Geometry: final body of the model. Coordinates: model frame, mm. A direction names the side the tool comes from. Coordinates: 2 decimals unless noted, no trailing zeros. Order: outer loops, then holes, each group sorted by start corner. A loop starts at its lowest first (then second) coordinate and runs counter-clockwise, first axis right, second up. Notation, with made-up numbers: (63.25, 54) - (86.25, 54) arc R13 ccw to (86.25, 73) - close; hole circle Ø11 at (45, 75.25). An arc over 180 degrees is marked (long way). Use a Markdown table: item, result. Add a question column.
```python
from build123d import *

# Parameters (mm, degrees)
SKETCH1_W                      = 174
SKETCH1_H                      = 50
BOSS_EXTRUDE1_DEPTH            = 13
M6_CLEARANCE_HOLE1_D           = 6.6
M6_CLEARANCE_HOLE1_CSINK_D     = 6.65
M6_CLEARANCE_HOLE1_CSINK_ANGLE = 100
SKETCH6_W                      = 80
SKETCH6_H                      = 13
BOSS_EXTRUDE2_DEPTH            = 40
SKETCH7_W                      = 80
SKETCH7_H                      = 40
BOSS_EXTRUDE3_DEPTH            = 50
CUT_EXTRUDE2_DEPTH             = 120.557517539
CUT_EXTRUDE2_DEPTH_BACK        = 120.557517539
SKETCH9_R                      = 14.29
M6_CLEARANCE_HOLE2_AT_2_COUNT  = 2
M6_CLEARANCE_HOLE2_AT_2_PITCH  = 37.540299013
M6_CLEARANCE_HOLE2_AT_3_COUNT  = 2
M6_CLEARANCE_HOLE2_AT_3_PITCH  = 37.540299013
M6_CLEARANCE_HOLE2_AT_4_COUNT  = 2
M6_CLEARANCE_HOLE2_AT_4_PITCH  = 53.09
CUT_EXTRUDE3_DEPTH             = 6.93
CUT_EXTRUDE3_DEPTH_BACK        = 6.93
SKETCH17_W                     = 28.58
SKETCH17_H                     = 29
CUT_EXTRUDE4_DEPTH             = 135.792433022
CUT_EXTRUDE5_DEPTH             = 50


with BuildPart() as part:
    # Sketch1 → Boss-Extrude1 (new body)
    with BuildSketch(Plane(origin=(0, 0, 0), x_dir=(1, 0, 0), z_dir=(0, 1, 0))):
        Rectangle(SKETCH1_W, SKETCH1_H)
    extrude(amount=BOSS_EXTRUDE1_DEPTH)

    # M6 Clearance Hole1 (through all)
    with Locations(Plane(origin=(0, 13, 0), x_dir=(1, 0, 0), z_dir=(0, 1, 0))):
        with Locations((-80, 20), (-40, 20), (-80, -20), (-40, -20), (40, 20), (80, 20), (40, -20), (80, -20)):
            CounterSinkHole(M6_CLEARANCE_HOLE1_D / 2, M6_CLEARANCE_HOLE1_CSINK_D / 2, counter_sink_angle=M6_CLEARANCE_HOLE1_CSINK_ANGLE)

    # Sketch6 → Boss-Extrude2 (add)
    with BuildSketch(Plane.XY.offset(25)):
        with Locations((0, 6.5)):
            Rectangle(SKETCH6_W, SKETCH6_H)
    extrude(amount=BOSS_EXTRUDE2_DEPTH)

    # Sketch7 → Boss-Extrude3 (add)
    with BuildSketch(Plane.XZ):
        with Locations((0, 45)):
            Rectangle(SKETCH7_W, SKETCH7_H)
    extrude(amount=BOSS_EXTRUDE3_DEPTH)

    # Sketch9 → Cut-Extrude2 (cut, two sides: drawn at the far end of the back side and taken through both)
    with BuildSketch(Plane.XY.offset(-CUT_EXTRUDE2_DEPTH_BACK)):
        with Locations((0, -21)):
            Circle(SKETCH9_R)
    extrude(amount=CUT_EXTRUDE2_DEPTH + CUT_EXTRUDE2_DEPTH_BACK, mode=Mode.SUBTRACT)

    # Sketch13 → M6 Clearance Hole2 (revolve, cut)
    with BuildSketch(Plane(origin=(-18.770149507, -2.229850493, 25), x_dir=(0, 1, 0), z_dir=(1, 0, 0))):
        Polygon((0, 0), (0, 40), (3.3, 40), (3.3, 0.020977491), (3.325, 0), align=None)
    m6_clearance_hole2 = revolve(axis=Axis((-18.770149507, -2.229850493, 18.65), (0, 0, 1)), mode=Mode.SUBTRACT)

    # M6 Clearance Hole2 at 2: M6 Clearance Hole2 ×2
    with Locations(*[(0, -i * M6_CLEARANCE_HOLE2_AT_2_PITCH, 0) for i in range(1, M6_CLEARANCE_HOLE2_AT_2_COUNT)]):
        add(m6_clearance_hole2, mode=Mode.SUBTRACT)

    # M6 Clearance Hole2 at 3: M6 Clearance Hole2 ×2
    with Locations(*[(i * M6_CLEARANCE_HOLE2_AT_3_PITCH, 0, 0) for i in range(1, M6_CLEARANCE_HOLE2_AT_3_COUNT)]):
        add(m6_clearance_hole2, mode=Mode.SUBTRACT)

    # M6 Clearance Hole2 at 4: M6 Clearance Hole2 ×2
    with Locations(*[Vector(0.7071067811865476, -0.7071067811865475, 0) * (i * M6_CLEARANCE_HOLE2_AT_4_PITCH) for i in range(1, M6_CLEARANCE_HOLE2_AT_4_COUNT)]):
        add(m6_clearance_hole2, mode=Mode.SUBTRACT)

    # Sketch16 → Cut-Extrude3 (cut, two sides: drawn at the far end of the back side and taken through both)
    with BuildSketch(Plane.XY.offset(45).offset(-CUT_EXTRUDE3_DEPTH_BACK)):
        with BuildLine():
            Line((-33.22, -21), (-33.22, -50))
            Line((-33.22, -50), (33.22, -50))
            Line((33.22, -50), (33.22, -21))
            ThreePointArc((33.22, -21), (0, 12.22), (-33.22, -21))
        make_face()
    extrude(amount=CUT_EXTRUDE3_DEPTH + CUT_EXTRUDE3_DEPTH_BACK, mode=Mode.SUBTRACT)

    # Sketch17 → Cut-Extrude4 (cut, through all)
    with BuildSketch(Plane.XY.offset(65)):
        with Locations((0, -35.5)):
            Rectangle(SKETCH17_W, SKETCH17_H)
    extrude(amount=-CUT_EXTRUDE4_DEPTH, mode=Mode.SUBTRACT)

    # Sketch19 → Cut-Extrude5 (cut)
    with BuildSketch(Plane(origin=(0, 0, -25), x_dir=(-1, 0, 0), z_dir=(0, 0, -1))):
        Polygon((-30.618301393, 0), (-24.118301393, 6.5), (24.118301393, 6.5), (30.618301393, 0), align=None)
    extrude(amount=-CUT_EXTRUDE5_DEPTH, mode=Mode.SUBTRACT)


solid = part.part
```
1) Line query: line 1 (X direction, y = 9.25, z = 20); line 2 (Z direction, x = -80, y = 5); line 3 (X direction, y = -37.5, z = 49). Output: solid intervals per line, ascending. Write a range as from..to.
2) Section query A-A (z = -20). Give the number of separate pieces and of enclosed holes in the cut face, and give its area (3 significant figures).
3) Draft query along Y for faces 1 (the flat face through (-1, -4, 65)), 2 (the cylindrical face through (22, -2.9, 31.5)), 3 (the flat face through (-36, -50, 45)). Return one class per face: released by +Y, released by -Y, zero draft, split by the parting line, or undercut.
4) Access query for faces 4 (the flat face through (-33.22, -35, 45)), 5 (the flat face through (-64, 6, 25)), 6 (the flat face through (-14.29, -36, 59)). Directions: +Z, -Z, +X, -X, +Y, -Y. A direction counts if a zero-diameter tool reaches every point of the face in a straight line with its end or side. Return the directions, or none.
5) First-contact query: pin 1 (4 mm diameter, centred on x = -56.5, y = 5.5, fed in from +Z); pin 2 (7.5 mm diameter, centred on x = -18.77, y = -2.23, fed in from -Z); pin 3 (3 mm diameter, centred on y = -25, z = 28, fed in from -X); pin 4 (4 mm diameter, centred on x = -40, z = -20, fed in from -Y) (3 decimals). Flat tips, straight axial feed; report the tip coordinate or a pass-through.
6) Section query D-D (z = -6.5). Return the cut outline in (x, y).
7) Section query B-B (x = 80). Return the cut outline in (y, z) (3 decimals).
8) Section query C-C (y = -30.5). Return the cut outline in (x, z), and give its area (3 significant figures).
From the geometry:
| question | item | result |
|---|---|---|
| 1 | line 1 | x = -87..-83.3, -76.7..-43.3, -36.7..36.7, 43.3..76.7, 83.3..87 |
| 1 | line 2 | z = -25..-23.3, -16.7..16.7, 23.3..25 |
| 1 | line 3 | x = -40..-33.22, 33.22..40 |
| 2 | separate pieces | 5 |
| 2 | enclosed holes | 0 |
| 2 | area | 1,560 mm^2 |
| 3 | face 1 | zero draft |
| 3 | face 2 | undercut |
| 3 | face 3 | released by -Y |
| 4 | face 4 | -Y |
| 4 | face 5 | +Z, -X, +Y, -Y |
| 4 | face 6 | +Z, -Z, -Y |
| 5 | pin 1 | stops at z = 25 |
| 5 | pin 2 | stops at z = 25 |
| 5 | pin 3 | stops at x = -40 |
| 5 | pin 4 | passes through |
| 6 | outline | (-87, 0) - (-30.62, 0) - (-24.12, 6.5) - (24.12, 6.5) - (30.62, 0) - (87, 0) - (87, 13) - (-87, 13) - close |
| 7 | outline | (0, -25) - (13, -25) - (13, -23.325) - (12.979, -23.3) - (0, -23.3) - close; (0, -16.7) - (12.979, -16.7) - (13, -16.675) - (13, 16.675) - (12.979, 16.7) - (0, 16.7) - close; (0, 23.3) - (12.979, 23.3) - (13, 23.325) - (13, 25) - (0, 25) - close |
| 8 | outline | (-40, 25) - (-14.29, 25) - (-14.29, 38.07) - (-33.22, 38.07) - (-33.22, 51.93) - (-14.29, 51.93) - (-14.29, 65) - (-40, 65) - close; (14.29, 25) - (40, 25) - (40, 65) - (14.29, 65) - (14.29, 51.93) - (33.22, 51.93) - (33.22, 38.07) - (14.29, 38.07) - close |
| 8 | area | 1,530 mm^2 |
